from build123d import *

# Parameters (mm, degrees)
MAIN_DEPTH              = 120
PERNO1_START            = 160
PERNO1_OUTLINE_R        = 51.5
PERNO1_DEPTH            = 80
PERNO1_2_OUTLINE_R      = 70
PERNO1_2_DEPTH          = 120
FILLET2_R               = 4
FILLET2_OF_MIRROR14_R   = 4
CHAMFER2_SIZE           = 5
PISTA_R                 = 17
CUT_EXTRUDE1_DEPTH      = 318.647603485
CUT_EXTRUDE1_DEPTH_BACK = 318.647603485
SKETCH12_W              = 447.780773858
SKETCH12_H              = 289.463518693


# Read off the part's stored shape, not the designer's step: Perno1
with BuildPart() as part:
    # MainBody → Main (new body)
    with BuildSketch(Plane(origin=(0, 0, 0), x_dir=(1, 0, 0), z_dir=(0, 1, 0))):
        Polygon((-110, 160), (110, 160), (170, 100), (170, -100), (110, -160), (-110, -160), (-170, -100), (-170, 100), align=None)
    extrude(amount=MAIN_DEPTH)

    # Perno1 outline → Perno1 (add)
    with BuildSketch(Plane.XY.offset(PERNO1_START)):
        with Locations((0, 60)):
            Circle(PERNO1_OUTLINE_R)
    perno1 = extrude(amount=PERNO1_DEPTH)

    # Perno1 2 outline → Perno1 2 (cut)
    with BuildSketch(Plane(origin=(0, 0, 0), x_dir=(1, 0, 0), z_dir=(0, 1, 0))):
        Circle(PERNO1_2_OUTLINE_R)
    perno1_2 = extrude(amount=PERNO1_2_DEPTH, mode=Mode.SUBTRACT)

    # Fillet2
    fillet2_edges = [part.edges().sort_by_distance(p)[0] for p in [
        (-51.5, 60, 160),
    ]]
    fillet(fillet2_edges, radius=FILLET2_R)

    # Mirror14: Perno1, Perno1 2 across plane
    add(perno1.mirror(Plane.XY))
    add(perno1_2.mirror(Plane.XY), mode=Mode.SUBTRACT)

    # Fillet2 of Mirror14
    fillet2_of_mirror14_edges = [part.edges().sort_by_distance(p)[0] for p in [
        (-51.5, 60, -160),
    ]]
    fillet(fillet2_of_mirror14_edges, radius=FILLET2_OF_MIRROR14_R)

    # Chamfer2
    chamfer2_edges = [part.edges().sort_by_distance(p)[0] for p in [
        (-70, 0, 0),
    ]]
    chamfer(chamfer2_edges, length=CHAMFER2_SIZE)

    # Pista → PistaCut (revolve, cut)
    with BuildSketch(Plane.XY, mode=Mode.PRIVATE) as pistacut_sk:
        with Locations((106, 128)):
            Circle(PISTA_R)
    revolve(pistacut_sk.sketch.rotate(Axis((0, 120, 0), (0, -1, 0)), 90), axis=Axis((0, 120, 0), (0, -1, 0)), mode=Mode.SUBTRACT)

    # Sketch12 → Cut-Extrude1 (cut, two sides: drawn at the far end of the back side and taken through both)
    with BuildSketch(Plane(origin=(0, 0, 0), x_dir=(1, 0, 0), z_dir=(0, 1, 0)).offset(-CUT_EXTRUDE1_DEPTH_BACK)):
        with Locations((7.371920004, 144.731759347)):
            Rectangle(SKETCH12_W, SKETCH12_H)
    extrude(amount=CUT_EXTRUDE1_DEPTH + CUT_EXTRUDE1_DEPTH_BACK, mode=Mode.SUBTRACT)


solid = part.part
Part model, mm, in its own coordinate system. A direction names the side the tool comes from. Give positions to 0.01 mm unless a question says otherwise; leave off trailing zeros. Loops run counter-clockwise (first coordinate to the right, second up) from the corner with the lowest first, then second, coordinate; pieces in that order, holes last.
(1) Band-saw the part on C-C (z = 127). Write the cut outline in (x, y).
Return value:
outline: (-143, 0) - (143, 0) - (143, 120) - (-143, 120) - close
(2) Pin check, flat tips, straight feed: pin 1 (1.5 mm diameter, centred on x = 75, y = 51.5, fed in from +Z); pin 2 (3 mm diameter, centred on y = 60.5, z = 196.5, fed in from +X); pin 3 (5 mm diameter, centred on y = 38, z = 184.5, fed in from -X). Stop position of each tip, or through.
Return value:
pin 1: stops at z = 160
pin 2: stops at x = 51.5
pin 3: stops at x = -47.67
(3) Drill centre lines: line 1 along X through (y, z) = (29.5, 34); line 2 along X through (y, z) = (56, 45); line 3 along Y through (x, z) = (30, 176). Where is each one in solid material? Low to high.
Return value:
line 1: x = -170 to -61.19, 61.19 to 170
line 2: x = -170 to -53.62, 53.62 to 170
line 3: y = 18.14 to 101.86
(4) Band-saw the part on A-A (y = 60). Write the cut outline in (x, z).
Return value:
outline: (-170, 0) - (-70, 0) arc R70 cw to (70, 0) - (170, 0) - (170, 100) - (110, 160) - (55.5, 160) arc R4 cw to (51.5, 164) - (51.5, 240) - (-51.5, 240) - (-51.5, 164) arc R4 cw to (-55.5, 160) - (-110, 160) - (-170, 100) - close
(5) 3-axis set-ups, long thin cutter, end or side, ignore diameter. For faces 4 (the flat face through (50, 86, 160)), 5 (the flat face through (140, 59, 130)): which of +Z, -Z, +X, -X, +Y, -Y reach the whole face in a straight line?
Return value:
face 4: +Z
face 5: +Z, +X, +Y, -Y
(6) Band-saw the part on B-B (x = 0). Write the cut outline in (y, z).
Return value:
outline: (0, 75) - (5, 70) - (120, 70) - (120, 91) arc R17 cw to (120, 121) - (120, 160) - (115.5, 160) arc R4 cw to (111.5, 164) - (111.5, 240) - (8.5, 240) - (8.5, 164) arc R4 cw to (4.5, 160) - (0, 160) - close
(7) Pull direction X, two halves, no side cores. Call faces 1 (the flat face through (2, 0, 79)), 2 (the flat face through (170, 59, 49)), 3 (the conical face through (-1.545, 4.757, 70.226)): pulls with the +X half, pulls with the -X half, needs draft (parallel to the pull), parting line crosses it, or undercut.
Return value:
face 1: needs draft
face 2: pulls with the +X half
face 3: undercut
